```python
from build123d import *

# Parameters (mm, degrees)
SKETCH1_R           = 2.38125
BOSS_EXTRUDE1_DEPTH = 3.175


with BuildPart() as part:
    # Sketch1 → Boss-Extrude1 (new body)
    with BuildSketch(Plane.XY):
        with BuildLine():
            Line((-381, 0), (381, 0))
            Line((381, 0), (381, 203.2))
            Line((381, 203.2), (330.2, 203.2))
            Line((330.2, 203.2), (330.2, 152.4))
            ThreePointArc((330.2, 152.4), (315.321024484, 116.478975516), (279.4, 101.6))
            Line((279.4, 101.6), (-279.4, 101.6))
            ThreePointArc((-279.4, 101.6), (-315.321024484, 116.478975516), (-330.2, 152.4))
            Line((-330.2, 152.4), (-330.2, 203.2))
            Line((-330.2, 203.2), (-381, 203.2))
            Line((-381, 203.2), (-381, 0))
        make_face()
        with Locations((-355.6, 152.4)):
            Circle(SKETCH1_R, mode=Mode.SUBTRACT)
        with Locations((355.6, 152.4)):
            Circle(SKETCH1_R, mode=Mode.SUBTRACT)
        with Locations((355.6, 101.6)):
            Circle(SKETCH1_R, mode=Mode.SUBTRACT)
        with Locations((355.6, 50.8)):
            Circle(SKETCH1_R, mode=Mode.SUBTRACT)
        with Locations((-355.6, 101.6)):
            Circle(SKETCH1_R, mode=Mode.SUBTRACT)
        with Locations((-355.6, 50.8)):
            Circle(SKETCH1_R, mode=Mode.SUBTRACT)
    extrude(amount=BOSS_EXTRUDE1_DEPTH)


solid = part.part
```
Check sheet for the modelled part. Datum: model origin and axes. Units: mm. A direction names the side the tool comes from. Round coordinates to 2 decimals unless told otherwise and drop trailing zeros. Order: outer loops, then holes, each group sorted by start corner. A loop starts at its lowest first (then second) coordinate and runs counter-clockwise, first axis right, second up. Notation, with made-up numbers: (33.5, -23) - (43.5, -23) arc R28 cw to (43.5, 5) - close; hole circle Ø3 at (85.25, 46.25). An arc over 180 degrees is marked (long way). Write item = value, one per line.
Q1. Go/stop test with flat-tipped pins: pin 1 (5.5 mm diameter, centred on x = -355.6, y = 152.4, fed in from +Z) (3 decimals); pin 2 (1.6 mm diameter, centred on x = 86.5, z = 1.5, fed in from +Y); pin 3 (3 mm diameter, centred on x = -355.6, y = 50.8, fed in from +Z). Record where each tip stops, or that it passes through.
Computed:
pin_1 = 3.175
pin_2 = 101.6
pin_3 = through
Q2. Thickness scan on line 1 along Y through (x, z) = (355.6, 1.55); line 2 along X through (y, z) = (152.4, 2.25); line 3 along X through (y, z) = (177.5, 2.4). Record the ranges inside material, lowest first.
Computed:
line_1 = 0 to 48.42, 53.18 to 99.22, 103.98 to 150.02, 154.78 to 203.2
line_2 = -381 to -357.98, -353.22 to -330.2, 330.2 to 353.22, 357.98 to 381
line_3 = -381 to -330.2, 330.2 to 381
Q3. Section check B-B (x = 40). Record the boundary of the cut face in (y, z) (3 decimals).
Computed:
outline = (0, 0) - (101.6, 0) - (101.6, 3.175) - (0, 3.175) - close
Q4. Tool access check on faces 3 (the face through (-5, 58, 0)), 4 (the face through (315.714, 116.876, 1.565)). Record the directions out of +Z, -Z, +X, -X, +Y, -Y that give a thin tool (end or side, any length) a straight path to the whole face; none if there is none.
Computed:
face_3 = -Z, +X, -X, +Y, -Y
face_4 = +Z, -Z, +Y
Q5. Section check A-A (z = 0.65). Record the boundary of the cut face in (x, y), and give its area (3 significant figures).
Computed:
outline = (-381, 0) - (381, 0) - (381, 203.2) - (330.2, 203.2) - (330.2, 152.4) arc R50.8 cw to (279.4, 101.6) - (-279.4, 101.6) arc R50.8 cw to (-330.2, 152.4) - (-330.2, 203.2) - (-381, 203.2) - close; hole circle Ø4.76 at (-355.6, 50.8); hole circle Ø4.76 at (-355.6, 101.6); hole circle Ø4.76 at (-355.6, 152.4); hole circle Ø4.76 at (355.6, 50.8); hole circle Ø4.76 at (355.6, 101.6); hole circle Ø4.76 at (355.6, 152.4)
area = 88,700 mm^2
Q6. Draft check along X on faces 1 (the face through (-5, 58, 3.175)), 2 (the face through (-314.924, 116.086, 1.565)). Enter one of: pulls with the +X half, pulls with the -X half, needs draft (parallel to the pull), parting line crosses it, or undercut.
Computed:
face_1 = needs draft
face_2 = undercut
